from build123d import *

# Parameters (mm, degrees)
EXTRUIR_L_MINA1_DEPTH = 20


with BuildPart() as part:
    # Croquis1 → Extruir-Lámina1 (new body, symmetric)
    with BuildSketch(Plane.XY):
        with BuildLine():
            Line((-18.897074708, 59.824622078), (-4.536226315, 39.360848393))
            ThreePointArc((-4.536226315, 39.360848393), (-1.161015729, 32.530128082), (0, 25))
            Line((0, 25), (0, 0))
            Line((0, 0), (-3.5, 0))
            Line((-3.5, 0), (-3.5, 25))
            ThreePointArc((-3.5, 25), (-4.498473527, 31.475910151), (-7.401154631, 37.350329618))
            Line((-7.401154631, 37.350329618), (-21.762003023, 57.814103303))
            Line((-21.762003023, 57.814103303), (-18.897074708, 59.824622078))
        make_face()
    extrude(amount=EXTRUIR_L_MINA1_DEPTH, both=True)


solid = part.part
The listing builds one solid part. Answer for the finished solid, in the listing's coordinates (mm). A direction names the side the tool comes from. Round coordinates to 2 decimals unless told otherwise and drop trailing zeros. Order: outer loops, then holes, each group sorted by start corner. A loop starts at its lowest first (then second) coordinate and runs counter-clockwise, first axis right, second up. Notation, with made-up numbers: (-20.5, -40) -> (33.5, -40) arc R23 ccw to (33.5, -18) -> close; hole circle Ø9 at (-24.75, 22.5). An arc over 180 degrees is marked (long way). One line per item, written item: value.
Item 1: For faces 1 (the flat face through (-3.5, 12, 0)), 2 (the flat face through (0, 13, 0)), determine the directions among +Z, -Z, +X, -X, +Y, -Y from which every point of the face is accessible in a straight line to the end or side of a thin tool.
Taken from the geometry:
face 1: +Z, -Z, -X, -Y
face 2: +Z, -Z, +X, +Y, -Y
Item 2: Find section A-A, the plane z = -4.5. Give the vertices of the cut face in (x, y).
Taken from the geometry:
outline: (-21.76, 57.81) -> (-7.4, 37.35) arc R21.5 cw to (-3.5, 25) -> (-3.5, 0) -> (0, 0) -> (0, 25) arc R25 ccw to (-4.54, 39.36) -> (-18.9, 59.82) -> close
Item 3: Straight lines are drawn through the part: L1, parallel to X at y = 17.5, z = 11; L2, parallel to X at y = 33.5, z = -13; L3, parallel to Y at x = -7.75, z = -4.5. For each, find the intervals that lie inside material, in ascending order.
Taken from the geometry:
L1: x = -3.5 to 0
L2: x = -5.25 to -1.49
L3: y = 37.85 to 43.94
Item 4: Find section C-C, the plane x = -12.25. Give the vertices of the cut face in (y, z).
Taken from the geometry:
outline: (44.26, -20) -> (50.35, -20) -> (50.35, 20) -> (44.26, 20) -> close
Item 5: Find section B-B, the plane y = 23. Give the vertices of the cut face in (x, z).
Taken from the geometry:
outline: (-3.5, -20) -> (0, -20) -> (0, 20) -> (-3.5, 20) -> close
Item 6: Given P1, Ø12, axis at x = -7, y = 22, coming from the +Z side; P2, Ø4, axis at x = -14.5, z = 6.5, coming from the -Y side; P3, Ø6, axis at y = 13.5, z = 12, coming from the -X side; P4, Ø6, axis at x = -9, z = -14, coming from the -Y side, each flat-ended and moving along its own axis, determine where each tip first touches the part or whether it passes through.
Taken from the geometry:
P1: stops at z = 20
P2: stops at y = 44.62
P3: stops at x = -3.5
P4: stops at y = 35.06
